from build123d import *

# Parameters (mm, degrees)
SKETCH1_R           = 40
BOSS_EXTRUDE2_DEPTH = 10
SKETCH4_R           = 2.5
CUT_EXTRUDE3_DEPTH  = 15.4
CIRPATTERN1_COUNT   = 6
SKETCH3_R           = 35
BOSS_EXTRUDE4_DEPTH = 14.4
SKETCH8_R           = 3
CUT_EXTRUDE4_DEPTH  = 10
CIRPATTERN2_COUNT   = 8


with BuildPart() as part:
    # Sketch1 → Boss-Extrude2 (new body, symmetric)
    with BuildSketch(Plane(origin=(0, 0, 0), x_dir=(0, 0, -1), z_dir=(1, 0, 0))):
        Circle(SKETCH1_R)
    extrude(amount=BOSS_EXTRUDE2_DEPTH, both=True)

    # Sketch4 → Cut-Extrude3 (cut)
    with BuildSketch(Plane(origin=(0, 40, 0), x_dir=(1, 0, 0), z_dir=(0, 1, 0))):
        Circle(SKETCH4_R)
    cut_extrude3 = extrude(amount=-CUT_EXTRUDE3_DEPTH, mode=Mode.SUBTRACT)

    # CirPattern1: Cut-Extrude3 ×6 about axis
    cirpattern1_axis = Axis((0, 0, 0), (1, 0, 0))
    for i in range(1, CIRPATTERN1_COUNT):
        add(cut_extrude3.rotate(cirpattern1_axis, i * 360 / CIRPATTERN1_COUNT), mode=Mode.SUBTRACT)

    # Sketch3 → Boss-Extrude4 (add)
    with BuildSketch(Plane.ZY.offset(10)):
        Circle(SKETCH3_R)
    extrude(amount=BOSS_EXTRUDE4_DEPTH)

    # Sketch8 → Cut-Extrude4 (cut)
    with BuildSketch(Plane(origin=(0, 35, 0), x_dir=(1, 0, 0), z_dir=(0, 1, 0))):
        with Locations((-17.4, 0)):
            Circle(SKETCH8_R)
    cut_extrude4 = extrude(amount=-CUT_EXTRUDE4_DEPTH, mode=Mode.SUBTRACT)

    # CirPattern2: Cut-Extrude4 ×8 about axis
    cirpattern2_axis = Axis((0, 0, 0), (1, 0, 0))
    for i in range(1, CIRPATTERN2_COUNT):
        add(cut_extrude4.rotate(cirpattern2_axis, i * 360 / CIRPATTERN2_COUNT), mode=Mode.SUBTRACT)


solid = part.part
Can you work these out from the model? Positions are in its coordinate system, mm. A direction names the side the tool comes from. Give positions to 0.01 mm unless a question says otherwise; leave off trailing zeros. Loops run counter-clockwise (first coordinate to the right, second up) from the corner with the lowest first, then second, coordinate; pieces in that order, holes last. Notation, with made-up numbers: M -38.5,8.5 L 0.5,8.5 A15 ccw 0.5,17.5 Z; hole C 15,30.5 d9. An arc over 180 degrees is marked long. One line per item, written item: value. Start each with the question number.
1) If we section it at C-C, the plane x = 0: Write out the boundary of the cut face in (y, z), and give its area (3 significant figures).
2) If we section it at D-D, the plane y = 33: Write out the boundary of the cut face in (x, z).
3) If I drill on line 1 (X direction, y = 32.75, z = 0); line 2 (X direction, y = -6, z = 37); line 3 (Y direction, x = -17, z = 19), over which ranges is the centre line in solid material (lowest first)? Write a range as [from, to].
4) Thinking about a two-plate mould opening in Y: for faces 1 (the face through (0, -24.6, 0)), 2 (the face through (-14.54, -30.07, 0.9)), 3 (the face through (-17.442, 17.648, -17.707)), which applies, +Y half, -Y half, draft (parallel to the pull), parting line (faces both ways), or undercut?
5) On a 3-axis mill with a long thin cutter (end or side, diameter ignored), from which of +Z, -Z, +X, -X, +Y, -Y can I reach the whole of each face in a straight line? I mean faces 4 (the face through (-14.63, 1.15, -30.07)), 5 (the face through (-0.03, 12.27, -21.32)), 6 (the face through (2.385, -32.408, 0.751)), 7 (the face through (-0.54, 32.41, 2.44)). Say none if no direction works.
6) I'm going to push flat-ended pins straight in: pin 1 (3.5 mm diameter, centred on x = -17.4, y = 0, fed in from +Z); pin 2 (1 mm diameter, centred on y = 30.5, z = -20, fed in from -X); pin 3 (3 mm diameter, centred on x = -1.5, z = -16, fed in from +Y). Where does each tip first touch, or does it pass through?
7) If we section it at A-A, the plane y = 0: Write out the boundary of the cut face in (x, z), and give its area (3 significant figures).
8) If we section it at B-B, the plane z = 0: Write out the boundary of the cut face in (x, y).
Completed:
1. outline: M -39.92,-2.5 A40 ccw -22.13,-33.32 L -14.47,-20.05 L -10.13,-22.55 L -17.8,-35.82 A40 ccw 17.8,-35.82 L 10.13,-22.55 L 14.47,-20.05 L 22.13,-33.32 A40 ccw 39.92,-2.5 L 24.6,-2.5 L 24.6,2.5 L 39.92,2.5 A40 ccw 22.13,33.32 L 14.47,20.05 L 10.13,22.55 L 17.8,35.82 A40 ccw -17.8,35.82 L -10.13,22.55 L -14.47,20.05 L -22.13,33.32 A40 ccw -39.92,2.5 L -24.6,2.5 L -24.6,-2.5 Z
1. area: 4,570 mm^2
2. outline: M -24.4,-11.66 L -10,-11.66 L -10,-22.61 L 10,-22.61 L 10,22.61 L -10,22.61 L -10,11.66 L -24.4,11.66 Z; hole C -17.4,0 d6; hole C 0,0 d5
3. line 1: x = [-24.4, -20.4], [-14.4, -2.5], [2.5, 10]
3. line 2: x = [-10, 10]
3. line 3: y = [-29.39, -23.2], [-16.36, 16.36], [23.2, 29.39]
4. face 1: -Y half
4. face 2: draft
4. face 3: undercut
5. face 4: -Z
5. face 5: none
5. face 6: -Y
5. face 7: +Y
6. pin 1: stops at z = 25
6. pin 2: stops at x = -10
6. pin 3: stops at y = 37.28
7. outline: M -24.4,-35 L -20.4,-35 L -20.4,-25 L -14.4,-25 L -14.4,-35 L -10,-35 L -10,-40 L 10,-40 L 10,40 L -10,40 L -10,35 L -14.4,35 L -14.4,25 L -20.4,25 L -20.4,35 L -24.4,35 Z
7. area: 2,490 mm^2
8. outline: M -24.4,-35 L -20.4,-35 L -20.4,-25 L -14.4,-25 L -14.4,-35 L -10,-35 L -10,-40 L -2.5,-40 L -2.5,-24.6 L 2.5,-24.6 L 2.5,-40 L 10,-40 L 10,40 L 2.5,40 L 2.5,24.6 L -2.5,24.6 L -2.5,40 L -10,40 L -10,35 L -14.4,35 L -14.4,25 L -20.4,25 L -20.4,35 L -24.4,35 Z
